Check sheet for the modelled part. Datum: model origin and axes. Units: mm. Face numbers are marked on the shaded views. A direction names the side the tool comes from. Round coordinates to 2 decimals unless told otherwise and drop trailing zeros. Write each loop counter-clockwise with the first axis right and the second up, starting at its lowest first coordinate (ties: lowest second). Pieces come first, ordered by that corner, then holes. Notation, with made-up numbers: M 32,5 L 68,5 A13 cw 68,25 Z; hole C -1.5,17.25 d3. An arc over 180 degrees is marked long. Put each result on its own line as item: value.
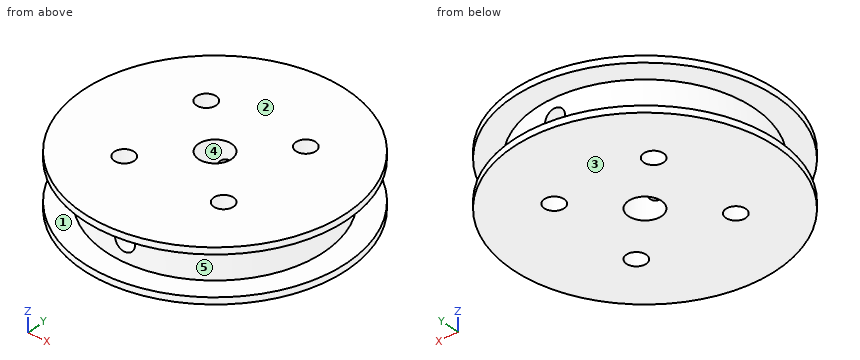
```python
from build123d import *

# Parameters (mm, degrees)
SKETCH1_R                                       = 20
PULLEY_BOSS_EXTRUDE1_DEPTH                      = 8
SKETCH2_W                                       = 3.5
SKETCH2_H                                       = 6
SKETCH3_R                                       = 2.5
SHAFT_CUT_EXTRUDE1_DEPTH                        = 8
SPRINT_HOLE_CUT_EXTRUDE2_REACH                  = 31.394
SPRINT_HOLE_CUT_EXTRUDE2_END_RADIUS             = 16.5
SKETCH4_R                                       = 1.5
SPRINT_HOLE_CUT_EXTRUDE2_DIRECTION_2_REACH      = 31.394
SPRINT_HOLE_CUT_EXTRUDE2_DIRECTION_2_END_RADIUS = 16.5
SKETCH5_R                                       = 1.5
ARM_DISTANS_MOUNTING_HOLES_CUT_EXTRUDE1_DEPTH   = 8


with BuildPart() as part:
    # Sketch1 → Pulley Boss-Extrude1 (new body)
    with BuildSketch(Plane.XY):
        Circle(SKETCH1_R)
    extrude(amount=PULLEY_BOSS_EXTRUDE1_DEPTH)

    # Sketch2 → Belt Cut-Revolve3 (revolve, cut)
    with BuildSketch(Plane(origin=(0, 0, 0), x_dir=(1, 0, 0), z_dir=(0, 1, 0)), mode=Mode.PRIVATE) as belt_cut_revolve3_sk:
        with Locations((18.25, -4)):
            Rectangle(SKETCH2_W, SKETCH2_H)
    revolve(belt_cut_revolve3_sk.sketch.rotate(Axis((0, 0, -14.62158436), (0, 0, 1)), 180), axis=Axis((0, 0, -14.62158436), (0, 0, 1)), mode=Mode.SUBTRACT)

    # Sketch3 → Shaft Cut-Extrude1 (cut)
    with BuildSketch(Plane.XY):
        Circle(SKETCH3_R)
    extrude(amount=SHAFT_CUT_EXTRUDE1_DEPTH, mode=Mode.SUBTRACT)

    # Sprint Hole Cut-Extrude2: up to this cylinder (the profile starts inside it)
    sprint_hole_cut_extrude2_end = Plane(origin=(0, 0, 4), z_dir=(0, 0, -1)) * Cylinder(SPRINT_HOLE_CUT_EXTRUDE2_END_RADIUS, 96.788, mode=Mode.PRIVATE)
    # Sketch4 → Sprint Hole Cut-Extrude2 (cut, up to the surface)
    with BuildSketch(Plane(origin=(0, 0, 0), x_dir=(1, 0, 0), z_dir=(0, 1, 0)), mode=Mode.PRIVATE) as sprint_hole_cut_extrude2_sk1:
        with Locations(Location((0, -4, 0), (0, 0, 270))):
            Circle(SKETCH4_R)
    sprint_hole_cut_extrude2_tool1 = extrude(sprint_hole_cut_extrude2_sk1.sketch, amount=-SPRINT_HOLE_CUT_EXTRUDE2_REACH, mode=Mode.PRIVATE) & sprint_hole_cut_extrude2_end
    add(sprint_hole_cut_extrude2_tool1.solids().sort_by_distance((0, 0, 4))[0], mode=Mode.SUBTRACT)

    # Sprint Hole Cut-Extrude2 direction 2: up to this cylinder (the profile starts inside it)
    sprint_hole_cut_extrude2_direction_2_end = Plane(origin=(0, 0, 4), z_dir=(0, 0, -1)) * Cylinder(SPRINT_HOLE_CUT_EXTRUDE2_DIRECTION_2_END_RADIUS, 96.788, mode=Mode.PRIVATE)
    # Sketch4 → Sprint Hole Cut-Extrude2 direction 2 (cut, up to the surface)
    with BuildSketch(Plane(origin=(0, 0, 0), x_dir=(1, 0, 0), z_dir=(0, 1, 0)), mode=Mode.PRIVATE) as sprint_hole_cut_extrude2_direction_2_sk1:
        with Locations(Location((0, -4, 0), (0, 0, 270))):
            Circle(SKETCH4_R)
    sprint_hole_cut_extrude2_direction_2_tool1 = extrude(sprint_hole_cut_extrude2_direction_2_sk1.sketch, amount=SPRINT_HOLE_CUT_EXTRUDE2_DIRECTION_2_REACH, mode=Mode.PRIVATE) & sprint_hole_cut_extrude2_direction_2_end
    add(sprint_hole_cut_extrude2_direction_2_tool1.solids().sort_by_distance((0, 0, 4))[0], mode=Mode.SUBTRACT)

    # Sketch5 → Arm Distans Mounting Holes Cut-Extrude1 (cut)
    with BuildSketch(Plane.XY.offset(8)):
        with Locations((7.5, 7.5)):
            Circle(SKETCH5_R)
        with Locations((-7.5, 7.5)):
            Circle(SKETCH5_R)
        with Locations((-7.5, -7.5)):
            Circle(SKETCH5_R)
        with Locations((7.5, -7.5)):
            Circle(SKETCH5_R)
    extrude(amount=-ARM_DISTANS_MOUNTING_HOLES_CUT_EXTRUDE1_DEPTH, mode=Mode.SUBTRACT)


solid = part.part
```
1. Depth check by flat-ended pin: pin 1 Ø2 at (y, z) = (10.5, 1) entering from -X; pin 2 Ø2.5 at (x, y) = (7.5, -7.5) entering from -Z; pin 3 Ø1.5 at (y, z) = (13, 3.5) entering from -X; pin 4 Ø1 at (x, z) = (-8.5, 4.5) entering from -Y. Enter the tip coordinate at first touch or a pass-through.
Computed values:
pin 1: stops at x = -17.6
pin 2: passes through
pin 3: stops at x = -11.05
pin 4: stops at y = -14.43
2. Cross-section at B-B (y = -6.5). Enter the section's corners in (x, z).
Computed values:
outline: M -18.91,0 L -8.62,0 L -8.62,8 L -18.91,8 L -18.91,7 L -15.17,7 L -15.17,1 L -18.91,1 Z; M -6.38,0 L 6.38,0 L 6.38,8 L -6.38,8 Z; M 8.62,0 L 18.91,0 L 18.91,1 L 15.17,1 L 15.17,7 L 18.91,7 L 18.91,8 L 8.62,8 Z; hole C 0,4 d3
3. Release check for a two-part mould opening along Z. For the marked faces 1, 2 and 3 record: +Z half, -Z half, draft (parallel to the pull), parting line (faces both ways), or undercut.
Computed values:
face 1: undercut
face 2: +Z half
face 3: -Z half
4. Cross-section at D-D (y = -13.5). Enter the section's corners in (x, z), then the cut area to 3 significant figures.
Computed values:
outline: M -14.76,0 L 14.76,0 L 14.76,1 L 9.49,1 L 9.49,7 L 14.76,7 L 14.76,8 L -14.76,8 L -14.76,7 L -9.49,7 L -9.49,1 L -14.76,1 Z; hole C 0,4 d3
area: 166 mm2
5. Scan lines: probe 1 along Y at (x, z) = (7.5, 3.5); probe 2 along Z at (x, y) = (0, -12.25); probe 3 along X at (y, z) = (-6.75, 4). Record each from-to range of solid material in increasing order.
Computed values:
probe 1: y = -14.7 to -9, -6 to 6, 9 to 14.7
probe 2: z = 0 to 2.5, 5.5 to 8
probe 3: x = -15.06 to -8.8, -6.2 to -1.5, 1.5 to 6.2, 8.8 to 15.06
6. Cross-section at A-A (x = 0). Enter the section's corners in (y, z), then the cut area to 3 significant figures.
Computed values:
outline: M -20,0 L -2.5,0 L -2.5,2.5 L -16.5,2.5 L -16.5,1 L -20,1 Z; M -20,7 L -16.5,7 L -16.5,5.5 L -2.5,5.5 L -2.5,8 L -20,8 Z; M 2.5,0 L 20,0 L 20,1 L 16.5,1 L 16.5,2.5 L 2.5,2.5 Z; M 2.5,5.5 L 16.5,5.5 L 16.5,7 L 20,7 L 20,8 L 2.5,8 Z
area: 154 mm2
7. Access from +Z, -Z, +X, -X, +Y, -Y to the whole of each face (thin tool, end or side, straight path). Record for the marked faces 4 and 5.
Computed values:
face 4: +Z, -Z
face 5: none
8. Cross-section at C-C (z = 4). Enter the section's corners in (x, y), then the cut area to 3 significant figures.
Computed values:
outline: M -1.5,-16.43 L -1.5,-2 A2.5 cw -1.5,2 L -1.5,16.43 A16.5 ccw Z; M 1.5,-16.43 A16.5 ccw 1.5,16.43 L 1.5,2 A2.5 cw 1.5,-2 Z; hole C -7.5,-7.5 d3; hole C -7.5,7.5 d3; hole C 7.5,-7.5 d3; hole C 7.5,7.5 d3
area: 723 mm2
